Geometry: final body of the model. Coordinates: model frame, mm. Face numbers are marked on the shaded views. A direction names the side the tool comes from. Give positions to 0.01 mm unless a question says otherwise; leave off trailing zeros. Loops run counter-clockwise (first coordinate to the right, second up) from the corner with the lowest first, then second, coordinate; pieces in that order, holes last.
from build123d import *

# Parameters (mm, degrees)
BOSS_EXTRUDE1_DEPTH                                  = 12.7
SKETCH2_R                                            = 31.75
BOSS_EXTRUDE2_DEPTH                                  = 38.1
CBORE_FOR_3_8_BINDING_HEAD_MACHINE_SCREW_D           = 38.1
CBORE_FOR_3_8_BINDING_HEAD_MACHINE_SCREW_CBORE_D     = 50.8
CBORE_FOR_3_8_BINDING_HEAD_MACHINE_SCREW_CBORE_DEPTH = 6.35
CBORE_FOR_3_8_BINDING_HEAD_MACHINE_S_2_D             = 10.16
CBORE_FOR_3_8_BINDING_HEAD_MACHINE_S_2_CBORE_D       = 16.002
CBORE_FOR_3_8_BINDING_HEAD_MACHINE_S_2_CBORE_DEPTH   = 3.302
SKETCH9_W                                            = 4.826
SKETCH9_H                                            = 38.1


with BuildPart() as part:
    # Sketch1 → Boss-Extrude1 (new body)
    with BuildSketch(Plane(origin=(0, 0, 0), x_dir=(1, 0, 0), z_dir=(0, 1, 0))):
        with BuildLine():
            Line((-52.614285714, 17.21182555), (-16.328571429, 34.423651101))
            ThreePointArc((-16.328571429, 34.423651101), (0, 38.1), (16.328571429, 34.423651101))
            Line((16.328571429, 34.423651101), (52.614285714, 17.21182555))
            ThreePointArc((52.614285714, 17.21182555), (63.5, 0), (52.614285714, -17.21182555))
            Line((52.614285714, -17.21182555), (16.328571429, -34.423651101))
            ThreePointArc((16.328571429, -34.423651101), (0, -38.1), (-16.328571429, -34.423651101))
            Line((-16.328571429, -34.423651101), (-52.614285714, -17.21182555))
            ThreePointArc((-52.614285714, -17.21182555), (-63.5, 0), (-52.614285714, 17.21182555))
        make_face()
    extrude(amount=BOSS_EXTRUDE1_DEPTH)

    # Sketch2 → Boss-Extrude2 (add)
    with BuildSketch(Plane(origin=(0, 12.7, 0), x_dir=(1, 0, 0), z_dir=(0, 1, 0))):
        with Locations(Location((0, 0, 0), (0, 0, 90))):
            Circle(SKETCH2_R)
    extrude(amount=BOSS_EXTRUDE2_DEPTH)

    # CBORE for 3_8 Binding Head Machine Screw (through all)
    with Locations(Plane(origin=(0, 50.8, 0), x_dir=(1, 0, 0), z_dir=(0, 1, 0))):
        with Locations((0, 0)):
            CounterBoreHole(CBORE_FOR_3_8_BINDING_HEAD_MACHINE_SCREW_D / 2, CBORE_FOR_3_8_BINDING_HEAD_MACHINE_SCREW_CBORE_D / 2, CBORE_FOR_3_8_BINDING_HEAD_MACHINE_SCREW_CBORE_DEPTH)

    # CBORE for 3_8 Binding Head Machine S 2 (through all)
    with Locations(Plane(origin=(0, 12.7, 0), x_dir=(1, 0, 0), z_dir=(0, 1, 0))):
        with Locations((-44.45, 0), (44.45, 0)):
            CounterBoreHole(CBORE_FOR_3_8_BINDING_HEAD_MACHINE_S_2_D / 2, CBORE_FOR_3_8_BINDING_HEAD_MACHINE_S_2_CBORE_D / 2, CBORE_FOR_3_8_BINDING_HEAD_MACHINE_S_2_CBORE_DEPTH)

    # Sketch9 → 3/8 (0.38) Diameter Hole1 (revolve, cut)
    with BuildSketch(Plane(origin=(0, 31.75, 0), x_dir=(0, 1, 0), z_dir=(1, 0, 0))):
        with Locations((2.413, 19.05)):
            Rectangle(SKETCH9_W, SKETCH9_H)
    revolve(axis=Axis((0, 31.75, -6.35), (0, 0, 1)), mode=Mode.SUBTRACT)


solid = part.part
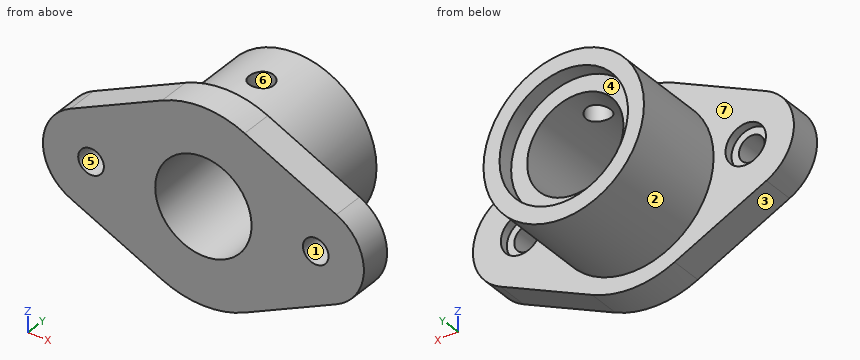
Item 1: Ray query, probe 1 along Y at (x, z) = (0, 24); probe 2 along Z at (x, y) = (11, 8); probe 3 along Y at (x, z) = (40.5, -9.5). Return the intervals inside material, ascending.
Values follow:
probe 1: y = 0 to 26.92, 36.58 to 44.45
probe 2: z = -36.48 to -15.55, 15.55 to 36.48
probe 3: y = 0 to 12.7
Item 2: Pin query (flat end, axial travel): pin 1 (5 mm diameter, centred on y = 6, z = -22, fed in from +X); pin 2 (4 mm diameter, centred on y = 6.5, z = 29, fed in from +X); pin 3 (9.5 mm diameter, centred on x = 44.45, z = 0, fed in from -Y); pin 4 (6 mm diameter, centred on x = 46, z = 5.5, fed in from +Y). Return the tip coordinate at first contact, or that it passes through.
Values follow:
pin 1: stops at x = 47.79
pin 2: stops at x = 31.98
pin 3: passes through
pin 4: stops at y = 12.7
Item 3: Section query C-C on y = 6.5. Return loops of the section in (x, z), plus the area to 3 significant figures.
Values follow:
outline: (-52.61, -17.21) - (-16.33, -34.42) arc R38.1 ccw to (16.33, -34.42) - (52.61, -17.21) arc R19.05 ccw to (52.61, 17.21) - (16.33, 34.42) arc R38.1 ccw to (-16.33, 34.42) - (-52.61, 17.21) arc R19.05 ccw to start; hole circle Ø10.16 at (-44.45, 0); hole circle Ø38.1 at (0, 0); hole circle Ø10.16 at (44.45, 0)
area: 5,390 mm2
Item 4: Set-up query: the marked faces 5, 6 and 7. Return all of +Z, -Z, +X, -X, +Y, -Y with unobstructed straight access to the full face (end or side cutting, diameter ignored); none if empty.
Values follow:
face 5: +Y, -Y
face 6: +Z
face 7: +Y
Item 5: Section query A-A on z = 0. Give the number of separate pieces and of enclosed holes in the cut face, plus the area to 3 significant figures.
Values follow:
separate pieces: 4
enclosed holes: 0
area: 1,720 mm2
Item 6: Section query D-D on z = -15.5. Return loops of the section in (x, y), plus the area to 3 significant figures.
Values follow:
outline: (-55.52, 0) - (-11.07, 0) - (-11.07, 44.45) - (-20.12, 44.45) - (-20.12, 50.8) - (-27.71, 50.8) - (-27.71, 12.7) - (-55.52, 12.7) - close; (11.07, 0) - (55.52, 0) - (55.52, 12.7) - (27.71, 12.7) - (27.71, 50.8) - (20.12, 50.8) - (20.12, 44.45) - (11.07, 44.45) - close
area: 2,280 mm2
Item 7: Section query B-B on x = 0. Return loops of the section in (y, z).
Values follow:
outline: (0, -38.1) - (12.7, -38.1) - (12.7, -31.75) - (50.8, -31.75) - (50.8, -25.4) - (44.45, -25.4) - (44.45, -19.05) - (0, -19.05) - close; (0, 19.05) - (26.92, 19.05) - (26.92, 31.75) - (12.7, 31.75) - (12.7, 38.1) - (0, 38.1) - close; (36.58, 19.05) - (44.45, 19.05) - (44.45, 25.4) - (50.8, 25.4) - (50.8, 31.75) - (36.58, 31.75) - close
Item 8: Draft query along X for the marked faces 1, 2, 3 and 4. Return one class per face: +X half, -X half, draft (parallel to the pull), parting line (faces both ways), or undercut.
Values follow:
face 1: undercut
face 2: parting line
face 3: -X half
face 4: undercut
